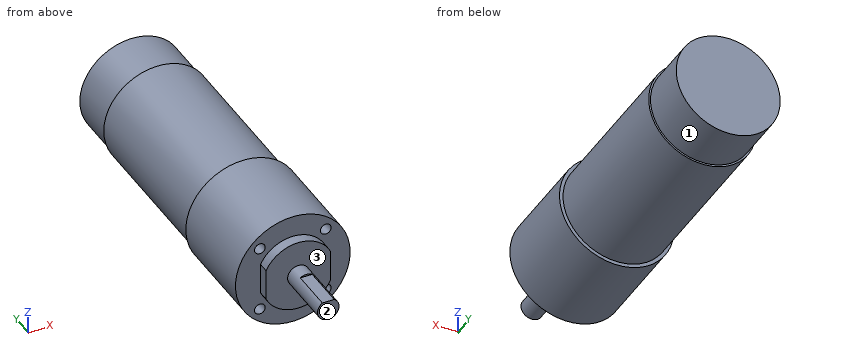
```python
from build123d import *

# Parameters (mm, degrees)
ESQUISSE1_R             = 16
EXTRUSION1_DEPTH        = 27
EXTRUSION2_DEPTH        = 3
ESQUISSE3_R             = 3
EXTRUSION3_DEPTH        = 16.3
ENL_V_MAT_EXTRU_1_DEPTH = 12
ESQUISSE5_R             = 15
EXTRUSION4_DEPTH        = 46.6
ESQUISSE6_R             = 1.5
ENL_V_MAT_EXTRU_2_DEPTH = 5.5
ESQUISSE7_R             = 14.5
EXTRUSION5_DEPTH        = 14


with BuildPart() as part:
    # Esquisse1 → Extrusion1 (new body)
    with BuildSketch(Plane(origin=(0, 0, 0), x_dir=(1, 0, 0), z_dir=(0, 1, 0))):
        Circle(ESQUISSE1_R)
    extrude(amount=EXTRUSION1_DEPTH)

    # Esquisse2 → Extrusion2 (add)
    with BuildSketch(Plane.XZ):
        with BuildLine():
            Line((-9, 4.358898944), (-9, -4.358898944))
            ThreePointArc((-9, -4.358898944), (0, -10), (9, -4.358898944))
            Line((9, -4.358898944), (9, 4.358898944))
            ThreePointArc((9, 4.358898944), (0, 10), (-9, 4.358898944))
        make_face()
    extrude(amount=EXTRUSION2_DEPTH)

    # Esquisse3 → Extrusion3 (add)
    with BuildSketch(Plane.XZ.offset(3)):
        Circle(ESQUISSE3_R)
    extrude(amount=EXTRUSION3_DEPTH)

    # Esquisse4 → Enlèv. mat.-Extru.1 (cut)
    with BuildSketch(Plane.XZ.offset(19.3)):
        with BuildLine():
            Line((-1.658312395, 2.5), (1.658312395, 2.5))
            ThreePointArc((1.658312395, 2.5), (0, 3), (-1.658312395, 2.5))
        make_face()
    extrude(amount=-ENL_V_MAT_EXTRU_1_DEPTH, mode=Mode.SUBTRACT)

    # Esquisse5 → Extrusion4 (add)
    with BuildSketch(Plane(origin=(0, 27, 0), x_dir=(-1, 0, 0), z_dir=(0, 1, 0))):
        Circle(ESQUISSE5_R)
    extrude(amount=EXTRUSION4_DEPTH)

    # Esquisse6 → Enlèv. mat.-Extru.2 (cut)
    with BuildSketch(Plane.XZ):
        with Locations((9.192388155, 9.192388155)):
            Circle(ESQUISSE6_R)
        with Locations((-9.192388155, 9.192388155)):
            Circle(ESQUISSE6_R)
        with Locations((9.192388155, -9.192388155)):
            Circle(ESQUISSE6_R)
        with Locations((-9.192388155, -9.192388155)):
            Circle(ESQUISSE6_R)
    extrude(amount=-ENL_V_MAT_EXTRU_2_DEPTH, mode=Mode.SUBTRACT)

    # Esquisse7 → Extrusion5 (add)
    with BuildSketch(Plane(origin=(0, 73.6, 0), x_dir=(-1, 0, 0), z_dir=(0, 1, 0))):
        Circle(ESQUISSE7_R)
    extrude(amount=EXTRUSION5_DEPTH)


solid = part.part
```
Build history of the part. All positions in model axes, mm. Face numbers are marked on the shaded views. A direction names the side the tool comes from. Round coordinates to 2 decimals unless told otherwise and drop trailing zeros. Loops run counter-clockwise (first coordinate to the right, second up) from the corner with the lowest first, then second, coordinate; pieces in that order, holes last.
Item 1: Saw through at A-A (z = 0). List the corners of the cut face in (x, y).
Item 2: Pin check, flat tips, straight feed: P1, Ø4, axis at x = -5, y = 60, coming from the +Z side; P2, Ø1.5, axis at x = 6, y = 22, coming from the -Z side; P3, Ø3, axis at y = 46, z = 9.5, coming from the +X side; P4, Ø4, axis at x = -10.5, y = -5.5, coming from the -Z side. Stop position of each tip, or through.
Item 3: Saw through at B-B (x = 0). List the corners of the cut face in (y, z), then the cut area to 3 significant figures.
Item 4: Saw through at D-D (z = -6). List the corners of the cut face in (x, y), then the cut area to 3 significant figures.
Item 5: Saw through at C-C (y = 68). List the corners of the cut face in (x, z).
Item 6: Which spindle directions (+Z, -Z, +X, -X, +Y, -Y) get a long thin tool onto all of the face, cutting with end or side? Do the marked faces 1, 2 and 3. Say none if no direction does.
Item 7: Drill centre lines: line 1 along Y through (x, z) = (11, 8); line 2 along Y through (x, z) = (-2.5, 9); line 3 along X through (y, z) = (80, -0.5). Where is each one in solid material? Low to high.
Worked answers:
1. outline: (-16, 0) - (-9, 0) - (-9, -3) - (-3, -3) - (-3, -19.3) - (3, -19.3) - (3, -3) - (9, -3) - (9, 0) - (16, 0) - (16, 27) - (15, 27) - (15, 73.6) - (14.5, 73.6) - (14.5, 87.6) - (-14.5, 87.6) - (-14.5, 73.6) - (-15, 73.6) - (-15, 27) - (-16, 27) - close
2. P1: stops at z = 14.7
2. P2: stops at z = -15.11
2. P3: stops at x = 12.69
2. P4: passes through
3. outline: (-19.3, -3) - (-3, -3) - (-3, -10) - (0, -10) - (0, -16) - (27, -16) - (27, -15) - (73.6, -15) - (73.6, -14.5) - (87.6, -14.5) - (87.6, 14.5) - (73.6, 14.5) - (73.6, 15) - (27, 15) - (27, 16) - (0, 16) - (0, 10) - (-3, 10) - (-3, 3) - (-7.3, 3) - (-7.3, 2.5) - (-19.3, 2.5) - close
3. area: 2,820 mm2
4. outline: (-14.83, 0) - (-8, 0) - (-8, -3) - (8, -3) - (8, 0) - (14.83, 0) - (14.83, 27) - (13.75, 27) - (13.75, 73.6) - (13.2, 73.6) - (13.2, 87.6) - (-13.2, 87.6) - (-13.2, 73.6) - (-13.75, 73.6) - (-13.75, 27) - (-14.83, 27) - close
4. area: 2,500 mm2
5. outline: circle Ø30 at (0, 0)
6. face 1: +Y
6. face 2: +Z, -Z, +X, -X, -Y
6. face 3: -Y
7. line 1: y = 0 to 87.6
7. line 2: y = -3 to 87.6
7. line 3: x = -14.49 to 14.49
